Read the model definition and answer for the solid it produces. Units are mm, in the model's axes. A direction names the side the tool comes from. Round coordinates to 2 decimals unless told otherwise and drop trailing zeros. Write each loop counter-clockwise with the first axis right and the second up, starting at its lowest first coordinate (ties: lowest second). Pieces come first, ordered by that corner, then holes. Notation, with made-up numbers: (-36.75, 64.5) - (-24.75, 64.5) arc R31 cw to (-24.75, 90.5) - close; hole circle Ø2 at (23.25, 55.25). An arc over 180 degrees is marked (long way). Use one line per item in the form item = value. Start each with the question number.
1) The part is cut by section C-C, the plane y = -0.5. Give the vertices of the cut face in (x, z).
2) The part is cut by section D-D, the plane z = -17.5. Give the vertices of the cut face in (x, y), plus the area to 3 significant figures.
3) For faces 1 (the face through (-5, 20, -17)), 2 (the face through (1, 0, 0)), determine the directions among +Z, -Z, +X, -X, +Y, -Y from which every point of the face is accessible in a straight line to the end or side of a thin tool.
4) Each of these flat-tipped pins is pushed along its axis until it touches: pin 1 (8 mm diameter, centred on x = 4, y = 12, fed in from -Z); pin 2 (10 mm diameter, centred on y = -8.5, z = -25, fed in from +X). Where does it stop, or does it pass through?
5) Consider line 1 along Y through (x, z) = (0.5, 1.8); line 2 along Z through (x, y) = (-2.25, -17); line 3 along X through (y, z) = (-7, -17). Determine where each line is inside the solid, lowest interval first. Write a range as from..to.
6) The part is cut by section A-A, the plane x = 2. Give the vertices of the cut face in (y, z).
7) For a pull along X with two mould halves and no side action, classify faces 3 (the face through (-4.5, 0, -25)), 4 (the face through (-0.04, -14.94, 1.52)), 5 (the face through (-7.5, 0, -23)), 6 (the face through (-6, 0, -50)) as released by +X, released by -X, zero draft, split by the parting line, or undercut.
8) The part is cut by section B-B, the plane y = -12.5. Give the vertices of the cut face in (x, z), plus the area to 3 significant figures.
from build123d import *

# Parameters (mm, degrees)
SKETCH1_W           = 15
SKETCH1_H           = 40
BOSS_EXTRUDE1_DEPTH = 3
SKETCH2_W           = 3
SKETCH2_H           = 40
BOSS_EXTRUDE2_DEPTH = 50
SKETCH3_R           = 2.5
CUT_EXTRUDE1_DEPTH  = 3
LPATTERN1_COUNT     = 2
LPATTERN1_PITCH     = 25


with BuildPart() as part:
    # Sketch1 → Boss-Extrude1 (new body)
    with BuildSketch(Plane.XY):
        Rectangle(SKETCH1_W, SKETCH1_H)
    extrude(amount=BOSS_EXTRUDE1_DEPTH)

    # Sketch2 → Boss-Extrude2 (add)
    with BuildSketch(Plane(origin=(0, 0, 0), x_dir=(-1, 0, 0), z_dir=(0, 0, -1))):
        with Locations((6, 0)):
            Rectangle(SKETCH2_W, SKETCH2_H)
    extrude(amount=BOSS_EXTRUDE2_DEPTH)

    # Sketch3 → Cut-Extrude1 (cut)
    with BuildSketch(Plane.XY.offset(3)):
        with Locations((0.5, 12.5)):
            Circle(SKETCH3_R)
    cut_extrude1 = extrude(amount=-CUT_EXTRUDE1_DEPTH, mode=Mode.SUBTRACT)

    # LPattern1: Cut-Extrude1 ×2
    with Locations(*[(0, -i * LPATTERN1_PITCH, 0) for i in range(1, LPATTERN1_COUNT)]):
        add(cut_extrude1, mode=Mode.SUBTRACT)


solid = part.part
Geometry results:
q1.outline = (-7.5, -50) - (-4.5, -50) - (-4.5, 0) - (7.5, 0) - (7.5, 3) - (-7.5, 3) - close
q2.outline = (-7.5, -20) - (-4.5, -20) - (-4.5, 20) - (-7.5, 20) - close
q2.area = 120 mm2
q3.face_1 = +Z, -Z, +X, -X, +Y
q3.face_2 = -Z, +X, +Y, -Y
q4.pin_1 = 0
q4.pin_2 = -4.5
q5.line_1 = -20..-15, -10..10, 15..20
q5.line_2 = 0..3
q5.line_3 = -7.5..-4.5
q6.outline = (-20, 0) - (-14.5, 0) - (-14.5, 3) - (-20, 3) - close; (-10.5, 0) - (10.5, 0) - (10.5, 3) - (-10.5, 3) - close; (14.5, 0) - (20, 0) - (20, 3) - (14.5, 3) - close
q7.face_3 = released by +X
q7.face_4 = undercut
q7.face_5 = released by -X
q7.face_6 = zero draft
q8.outline = (-7.5, -50) - (-4.5, -50) - (-4.5, 0) - (-2, 0) - (-2, 3) - (-7.5, 3) - close; (3, 0) - (7.5, 0) - (7.5, 3) - (3, 3) - close
q8.area = 180 mm2
